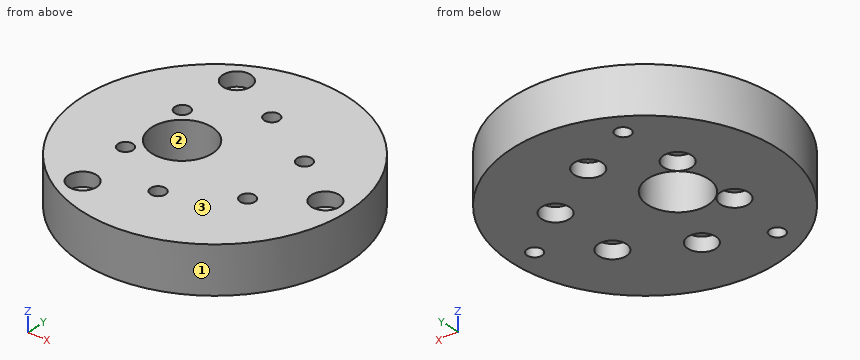
```python
from build123d import *

# Parameters (mm, degrees)
CROQUIS1_R              = 28.5
CROQUIS1_R_2            = 6.5
SALIENTE_EXTRUIR1_DEPTH = 10
MATRIZC2_COUNT          = 3
MATRIZC3_COUNT          = 6


with BuildPart() as part:
    # Croquis1 → Saliente-Extruir1 (new body)
    with BuildSketch(Plane.XY):
        Circle(CROQUIS1_R)
        with Locations((-7, 0)):
            Circle(CROQUIS1_R_2, mode=Mode.SUBTRACT)
    extrude(amount=SALIENTE_EXTRUIR1_DEPTH)

    # Croquis4 → Refrentado para tornillo con cabeza tron (revolve, cut)
    with BuildSketch(Plane(origin=(23.5, 0, 10), x_dir=(0, -1, 0), z_dir=(1, 0, 0))):
        Polygon((0, 0), (0, 20.96137699), (1.6, 20), (1.6, 3), (3, 3), (3, 0), align=None)
    refrentado_para_tornillo_con_cabeza_tron = revolve(axis=Axis((23.5, 0, 16.35), (0, 0, -1)), mode=Mode.SUBTRACT)

    # MatrizC2: Refrentado para tornillo con cabeza tron ×3 about axis
    matrizc2_axis = Axis((0, 0, 0), (0, 0, 1))
    for i in range(1, MATRIZC2_COUNT):
        add(refrentado_para_tornillo_con_cabeza_tron.rotate(matrizc2_axis, i * 360 / MATRIZC2_COUNT), mode=Mode.SUBTRACT)

    # Croquis9 → Refrentado para tornillo con cabeza  2 (revolve, cut)
    with BuildSketch(Plane(origin=(12.990381057, 7.5, 0), x_dir=(0, 1, 0), z_dir=(1, 0, 0))):
        Polygon((0, 0), (0, 20.96137699), (1.6, 20), (1.6, 3), (3, 3), (3, 0), align=None)
    refrentado_para_tornillo_con_cabeza_2 = revolve(axis=Axis((12.990381057, 7.5, -6.35), (0, 0, 1)), mode=Mode.SUBTRACT)

    # MatrizC3: Refrentado para tornillo con cabeza  2 ×6 about axis
    matrizc3_axis = Axis((0, 0, 0), (0, 0, 1))
    for i in range(1, MATRIZC3_COUNT):
        add(refrentado_para_tornillo_con_cabeza_2.rotate(matrizc3_axis, i * 360 / MATRIZC3_COUNT), mode=Mode.SUBTRACT)


solid = part.part
```
Source: CAD feature listing. Evaluate the final solid. Frame: model axes, mm. Face numbers are marked on the shaded views. Round coordinates to 2 decimals unless told otherwise and drop trailing zeros. Loops run counter-clockwise (first coordinate to the right, second up) from the corner with the lowest first, then second, coordinate; pieces in that order, holes last.
(1) Material intervals for probe 1 along X at (y, z) = (-7.5, 2); probe 2 along X at (y, z) = (-8.5, 6.25); probe 3 along Z at (x, y) = (11, -5.5), sorted ascending.
From the geometry:
probe 1: x = -27.5 to -15.99, -9.99 to 9.99, 15.99 to 27.5
probe 2: x = -27.2 to -14.24, -11.74 to 11.74, 14.24 to 27.2
probe 3: z = 3 to 10
(2) Section query A-A (x = -7). Output: boundary loops of the cut face in (y, z).
From the geometry:
outline: (-27.63, 0) - (-6.5, 0) - (-6.5, 10) - (-27.63, 10) - close; (6.5, 0) - (27.63, 0) - (27.63, 10) - (6.5, 10) - close
(3) Contact query for flat-ended pins moving along their axis: pin 1 Ø2.5 at (x, y) = (12.99, 7.5) entering from +Z; pin 2 Ø1.8 at (x, y) = (-1, -15.5) entering from -Z; pin 3 Ø1 at (y, z) = (-16.5, 4) entering from +X; pin 4 Ø1.5 at (y, z) = (-22, 3.5) entering from -X. Output: stop coordinate, or through.
From the geometry:
pin 1: passes through
pin 2: stops at z = 3
pin 3: stops at x = 23.58
pin 4: stops at x = -18.99
(4) Section query C-C (z = 5.25). Give the number of separate pieces and of enclosed holes in the cut face, and give its area (3 significant figures).
From the geometry:
separate pieces: 1
enclosed holes: 10
area: 2,350 mm2
(5) Section query B-B (y = -8). Output: boundary loops of the cut face in (x, z).
From the geometry:
outline: (-27.35, 0) - (-15.95, 0) - (-15.95, 3) - (-14.51, 3) - (-14.51, 10) - (-27.35, 10) - close; (-11.47, 3) - (-10.03, 3) - (-10.03, 0) - (10.03, 0) - (10.03, 3) - (11.47, 3) - (11.47, 10) - (-11.47, 10) - close; (14.51, 3) - (15.95, 3) - (15.95, 0) - (27.35, 0) - (27.35, 10) - (14.51, 10) - close
(6) Pull-direction query (X, two-part tool) for the marked faces 1, 2 and 3; classes: +X half, -X half, draft (parallel to the pull), parting line (faces both ways), or undercut.
From the geometry:
face 1: parting line
face 2: undercut
face 3: draft
(7) Section query D-D (y = 15). Output: boundary loops of the cut face in (x, z).
From the geometry:
outline: (-24.23, 0) - (-3, 0) - (-3, 3) - (-1.6, 3) - (-1.6, 10) - (-24.23, 10) - close; (1.6, 3) - (3, 3) - (3, 0) - (24.23, 0) - (24.23, 10) - (1.6, 10) - close
